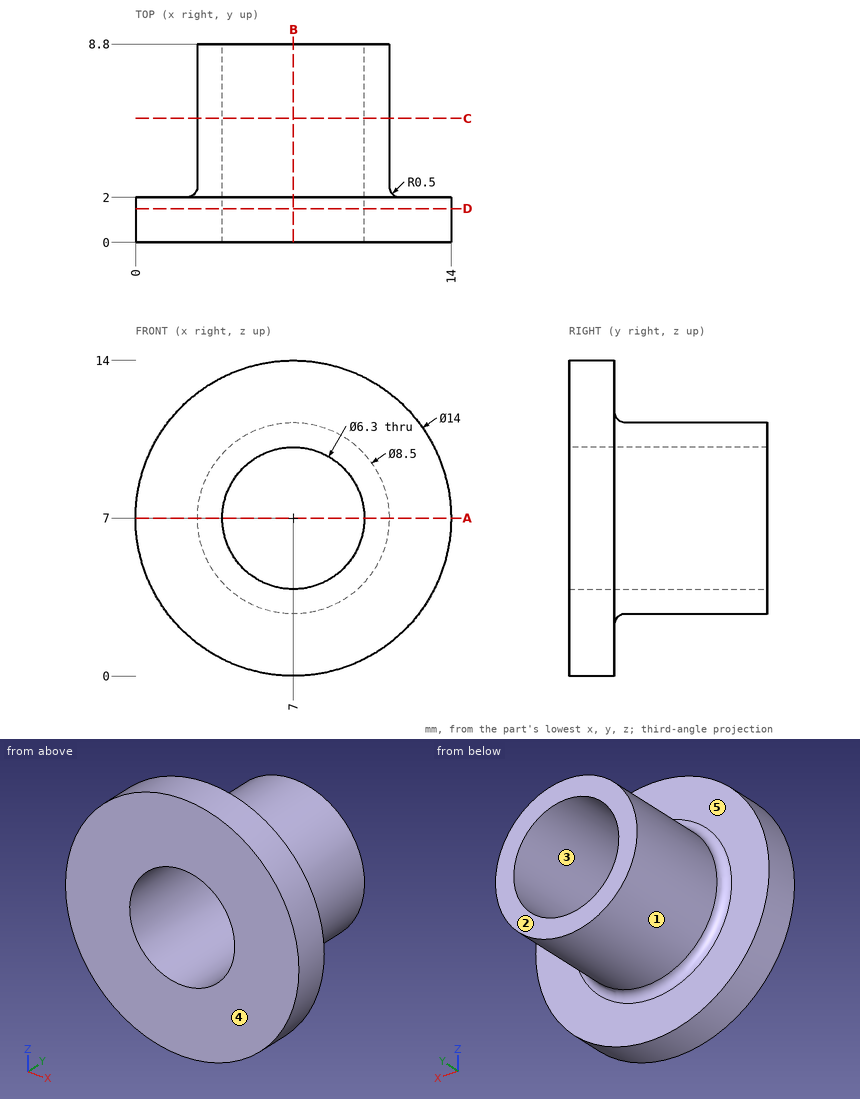
Verification items for this drawing (mm, ordinates from the low corner). A direction names the side the tool comes from. Round coordinates to 2 decimals unless told otherwise and drop trailing zeros. Loops run counter-clockwise (first coordinate to the right, second up) from the corner with the lowest first, then second, coordinate; pieces in that order, holes last. Notation, with made-up numbers: (15.25, -5.5) - (22.25, -5.5) arc R23 ccw to (22.25, 5.5) - close; hole circle Ø3 at (73.5, 55.5). An arc over 180 degrees is marked (long way). Answer as CSV lines item,"result". Start each with the question number.
Item 1: Section check C-C (y = 5.5). Record the boundary of the cut face in (x, z), and give its area (3 significant figures).
Item 2: Section check A-A (z = 7). Record the boundary of the cut face in (x, y).
Item 3: Set-up check for the marked faces 4 and 5: record each of +Z, -Z, +X, -X, +Y, -Y from which the full face is reachable in a straight line by a thin tool's end or side.
Item 4: Section check D-D (y = 1.5). Record the boundary of the cut face in (x, z).
Item 5: Depth check by flat-ended pin: P1, Ø3, axis at y = 6.5, z = 6, coming from the -X side; P2, Ø1.5, axis at x = 6, y = 4.5, coming from the +Z side; P3, Ø1, axis at x = 6.5, y = 6, coming from the -Z side. Enter the tip coordinate at first touch or a pass-through.
Item 6: Section check B-B (x = 7). Record the boundary of the cut face in (y, z).
Item 7: Scan lines: line 1 (X direction, y = 4, z = 7); line 2 (Y direction, x = 6.25, z = 11.25); line 3 (Y direction, x = 1.75, z = 11). Record each from-to range of solid material in increasing order. Write a range as [from, to].
Item 8: Release check for a two-part mould opening along X. For the marked faces 1, 2 and 3 record: +X half, -X half, draft (parallel to the pull), parting line (faces both ways), or undercut.
Report:
1,outline,"circle Ø8.5 at (7, 7); hole circle Ø6.3 at (7, 7)"
1,area,"25.6 mm2"
2,outline,"(0, 0) - (3.85, 0) - (3.85, 8.8) - (2.75, 8.8) - (2.75, 2.5) arc R0.5 cw to (2.25, 2) - (0, 2) - close; (10.15, 0) - (14, 0) - (14, 2) - (11.75, 2) arc R0.5 cw to (11.25, 2.5) - (11.25, 8.8) - (10.15, 8.8) - close"
3,face 4,"+Z, -Z, +X, -X, -Y"
3,face 5,"+Y"
4,outline,"circle Ø14 at (7, 7); hole circle Ø6.3 at (7, 7)"
5,P1,"stops at x = 2.75"
5,P2,"stops at z = 11.24"
5,P3,"stops at z = 2.75"
6,outline,"(0, 0) - (2, 0) - (2, 2.25) arc R0.5 cw to (2.5, 2.75) - (8.8, 2.75) - (8.8, 3.85) - (0, 3.85) - close; (0, 10.15) - (8.8, 10.15) - (8.8, 11.25) - (2.5, 11.25) arc R0.5 cw to (2, 11.75) - (2, 14) - (0, 14) - close"
7,line 1,"x = [2.75, 3.85], [10.15, 11.25]"
7,line 2,"y = [0, 2.25]"
7,line 3,"y = [0, 2]"
8,face 1,"parting line"
8,face 2,"draft"
8,face 3,"undercut"
